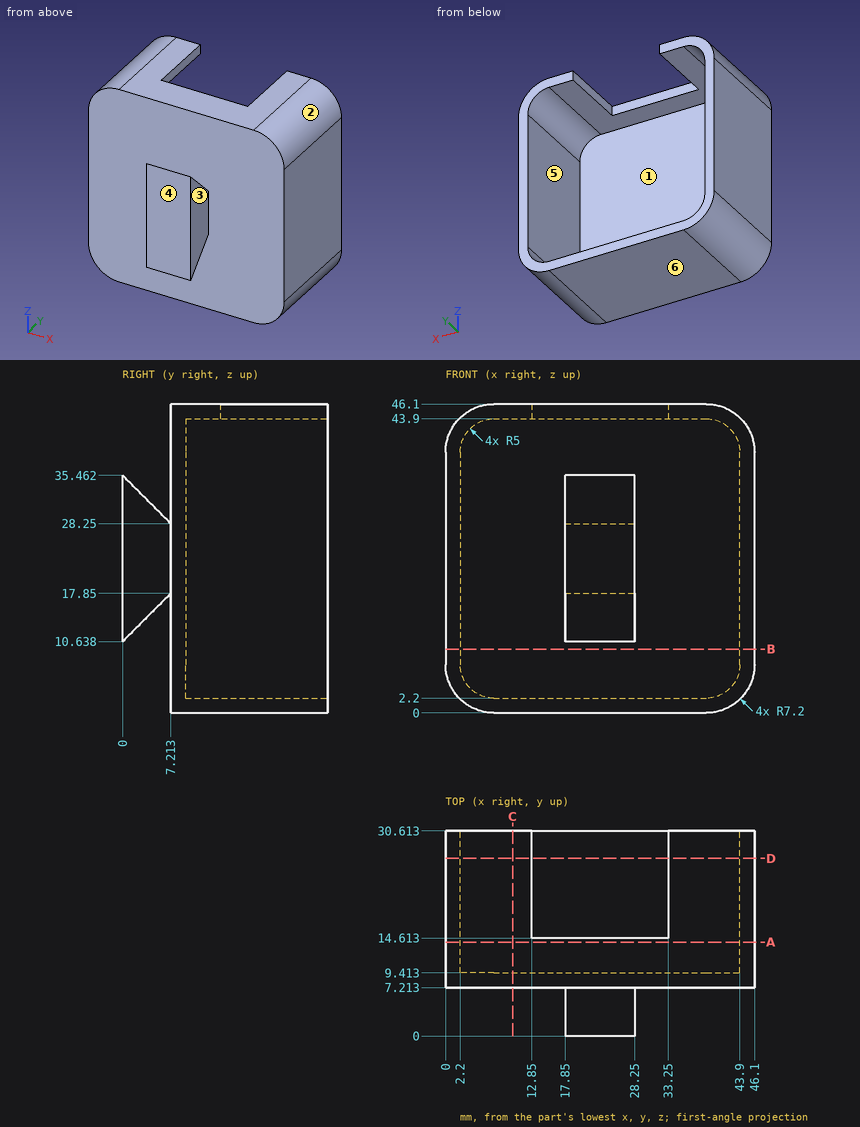
The drawing under review shows one solid part. Ordinate dimensions are in mm from its lowest x, y, z. A direction names the side the tool comes from. Round coordinates to 2 decimals unless told otherwise and drop trailing zeros. Write each loop counter-clockwise with the first axis right and the second up, starting at its lowest first coordinate (ties: lowest second). Pieces come first, ordered by that corner, then holes. Notation, with made-up numbers: (49, 72) -> (94, 72) arc R29 cw to (94, 101) -> close; hole circle Ø9 at (83.5, 31). An arc over 180 degrees is marked (long way). One line per question, with ' | ' between items. Start each with the question number.
(1) Insertion check: P1, Ø1.1, axis at y = 26, z = 45, coming from the +X side (1 decimal); P2, Ø6.5, axis at x = 20, y = 21, coming from the +Z side; P3, Ø3.5, axis at y = 4, z = 24, coming from the +X side. Each pin has a flat end and moves straight along its axis. Give the tip position at first contact, or say it passes through.
(2) Mouldability with a two-part tool opening along Z and no side actions: class the marked faces 4, 5 and 6 as released by +Z, released by -Z, zero draft, split by the parting line, or undercut.
(3) Add section B-B, the plane z = 9.5. Write out the cut boundary in (x, y).
(4) For line 1 along X through (y, z) = (28.5, 19); line 2 along Y through (x, z) = (17, 12), list the stretches that pass through material, from the lowest coordinate up. Write a range as from..to.
(5) Tool access review of the marked faces 1, 2 and 3: name each direction out of +Z, -Z, +X, -X, +Y, -Y from which nothing blocks a thin tool from reaching the whole face with its end or side.
(6) Add section C-C, the plane x = 10. Write out the cut boundary in (y, z), plus the area to 3 significant figures.
(7) Add section A-A, the plane y = 14. Write out the cut boundary in (x, z).
(8) Add section D-D, the plane y = 26.5. Write out the cut boundary in (x, z).
Answer list:
1) P1: x = 43.5 | P2: z = 2.2 | P3: x = 28.25
2) face 4: zero draft | face 5: undercut | face 6: released by -Z
3) outline: (0, 7.21) -> (46.1, 7.21) -> (46.1, 30.61) -> (43.9, 30.61) -> (43.9, 9.41) -> (2.2, 9.41) -> (2.2, 30.61) -> (0, 30.61) -> close
4) line 1: 0..2.2, 43.9..46.1 | line 2: 7.21..9.41
5) face 1: +Y | face 2: +Z, +X, +Y, -Y | face 3: +Z, -Z, +X, -Y
6) outline: (7.21, 0) -> (30.61, 0) -> (30.61, 2.2) -> (9.41, 2.2) -> (9.41, 43.9) -> (30.61, 43.9) -> (30.61, 46.1) -> (7.21, 46.1) -> close | area: 195 mm²
7) outline: (0, 7.2) arc R7.2 ccw to (7.2, 0) -> (38.9, 0) arc R7.2 ccw to (46.1, 7.2) -> (46.1, 38.9) arc R7.2 ccw to (38.9, 46.1) -> (7.2, 46.1) arc R7.2 ccw to (0, 38.9) -> close; hole (2.2, 7.2) arc R5 ccw to (7.2, 2.2) -> (38.9, 2.2) arc R5 ccw to (43.9, 7.2) -> (43.9, 38.9) arc R5 ccw to (38.9, 43.9) -> (7.2, 43.9) arc R5 ccw to (2.2, 38.9) -> close
8) outline: (0, 7.2) arc R7.2 ccw to (7.2, 0) -> (38.9, 0) arc R7.2 ccw to (46.1, 7.2) -> (46.1, 38.9) arc R7.2 ccw to (38.9, 46.1) -> (33.25, 46.1) -> (33.25, 43.9) -> (38.9, 43.9) arc R5 cw to (43.9, 38.9) -> (43.9, 7.2) arc R5 cw to (38.9, 2.2) -> (7.2, 2.2) arc R5 cw to (2.2, 7.2) -> (2.2, 38.9) arc R5 cw to (7.2, 43.9) -> (12.85, 43.9) -> (12.85, 46.1) -> (7.2, 46.1) arc R7.2 ccw to (0, 38.9) -> close
